from build123d import *

# Parameters (mm, degrees)
BOSS_EXTRUDE2_DEPTH     = 203.2
FILLET4_R               = 1.44
SKETCH3_R               = 1.61
SKETCH3_R_2             = 1.735
CUT_EXTRUDE2_DEPTH      = 1
CUT_EXTRUDE2_DEPTH_BACK = 16.14


with BuildPart() as part:
    # Sketch1 → Boss-Extrude2 (new body)
    with BuildSketch(Plane(origin=(0, 0, 0), x_dir=(0, 0, -1), z_dir=(1, 0, 0))):
        with BuildLine():
            Line((-10.98, 12.11), (-10.98, 1.44))
            ThreePointArc((-10.98, 1.44), (-10.558233765, 0.421766235), (-9.54, 0))
            Line((-9.54, 0), (9.54, 0))
            ThreePointArc((9.54, 0), (10.558233765, 0.421766235), (10.98, 1.44))
            Line((10.98, 1.44), (10.98, 12.11))
            ThreePointArc((10.98, 12.11), (11.401766235, 13.128233765), (12.42, 13.55))
            Line((12.42, 13.55), (18.85, 13.55))
            Line((18.85, 13.55), (18.85, 15.14))
            Line((18.85, 15.14), (10.83, 15.14))
            ThreePointArc((10.83, 15.14), (9.811766235, 14.718233765), (9.39, 13.7))
            Line((9.39, 13.7), (9.39, 3.03))
            ThreePointArc((9.39, 3.03), (8.968233765, 2.011766235), (7.95, 1.59))
            Line((7.95, 1.59), (-7.95, 1.59))
            ThreePointArc((-7.95, 1.59), (-8.968233765, 2.011766235), (-9.39, 3.03))
            Line((-9.39, 3.03), (-9.39, 13.7))
            ThreePointArc((-9.39, 13.7), (-9.811766235, 14.718233765), (-10.83, 15.14))
            Line((-10.83, 15.14), (-18.85, 15.14))
            Line((-18.85, 15.14), (-18.85, 13.55))
            Line((-18.85, 13.55), (-12.42, 13.55))
            ThreePointArc((-12.42, 13.55), (-11.401766235, 13.128233765), (-10.98, 12.11))
        make_face()
    extrude(amount=-BOSS_EXTRUDE2_DEPTH)

    # Fillet4
    fillet4_edges = [part.edges().sort_by_distance(p)[0] for p in [
        (0, 14.345, 18.85),
        (0, 14.345, -18.85),
        (-203.2, 14.345, 18.85),
        (-203.2, 14.345, -18.85),
    ]]
    fillet(fillet4_edges, radius=FILLET4_R)

    # Sketch3 → Cut-Extrude2 (cut, two sides)
    with BuildSketch(Plane(origin=(0, 15.14, 0), x_dir=(1, 0, 0), z_dir=(0, 1, 0))) as cut_extrude2_sk:
        with Locations((-101.6, 0)):
            Circle(SKETCH3_R)
        with Locations((-26.27, 0)):
            Circle(SKETCH3_R_2)
        with Locations((-176.93, 0)):
            Circle(SKETCH3_R_2)
        with Locations((-195.11, 14.89)):
            Circle(SKETCH3_R)
        with Locations((-195.11, -14.89)):
            Circle(SKETCH3_R)
        with Locations((-8.09, 14.89)):
            Circle(SKETCH3_R)
        with Locations((-8.09, -14.89)):
            Circle(SKETCH3_R)
        with BuildLine():
            Line((-137.43, -16.95), (-137.43, -18.85))
            Line((-137.43, -18.85), (-140.93, -18.85))
            Line((-140.93, -18.85), (-140.93, -16.95))
            ThreePointArc((-140.93, -16.95), (-139.18, -15.2), (-137.43, -16.95))
        make_face()
        with BuildLine():
            Line((-140.93, 18.85), (-140.93, 16.95))
            ThreePointArc((-140.93, 16.95), (-139.18, 15.2), (-137.43, 16.95))
            Line((-137.43, 16.95), (-137.43, 18.85))
            Line((-137.43, 18.85), (-140.93, 18.85))
        make_face()
        with BuildLine():
            Line((-65.77, -16.95), (-65.77, -18.85))
            Line((-65.77, -18.85), (-62.27, -18.85))
            Line((-62.27, -18.85), (-62.27, -16.95))
            ThreePointArc((-62.27, -16.95), (-64.02, -15.2), (-65.77, -16.95))
        make_face()
        with BuildLine():
            Line((-65.77, 16.95), (-65.77, 18.85))
            Line((-65.77, 18.85), (-62.27, 18.85))
            Line((-62.27, 18.85), (-62.27, 16.95))
            ThreePointArc((-62.27, 16.95), (-64.02, 15.2), (-65.77, 16.95))
        make_face()
    extrude(amount=CUT_EXTRUDE2_DEPTH, mode=Mode.SUBTRACT)
    extrude(cut_extrude2_sk.sketch, amount=-CUT_EXTRUDE2_DEPTH_BACK, mode=Mode.SUBTRACT)


solid = part.part
Verification items for the finished model (mm, model axes). A direction names the side the tool comes from. Give positions to 0.01 mm unless a question says otherwise; leave off trailing zeros. Order: outer loops, then holes, each group sorted by start corner. A loop starts at its lowest first (then second) coordinate and runs counter-clockwise, first axis right, second up. Notation, with made-up numbers: M -8.75,-24.5 L 11.25,-24.5 A19 cw 11.25,-0.5 Z; hole C 46.25,60 d8. An arc over 180 degrees is marked long. Use one line per item in the form item = value. Start each with the question number.
Q1. Mould release check, pull along X, two halves, no side actions. Record for faces 1 (the flat face through (-100, 15.14, -15)), 2 (the cylindrical face through (-196.72, 14.36, 14.82)), 3 (the flat face through (0, 1, 0)): +X half, -X half, draft (parallel to the pull), parting line (faces both ways), or undercut.
Q2. Section check B-B (x = -176.93). Enter the section's corners in (y, z) (3 decimals).
Q3. Go/stop test with flat-tipped pins: pin 1 Ø5.5 at (x, z) = (-26.27, 0) entering from +Y; pin 2 Ø5 at (x, z) = (-62, 15.5) entering from -Y; pin 3 Ø0.8 at (y, z) = (14, -18) entering from +X. Record where each tip stops, or that it passes through.
Q4. Scan lines: line 1 along X through (y, z) = (0.75, 0) (3 decimals); line 2 along X through (y, z) = (14.15, 14.89); line 3 along Z through (x, y) = (-26.27, 0.8) (3 decimals). Record each from-to range of solid material in increasing order. Write a range as [from, to].
Q5. Section check A-A (y = 8). Enter the section's corners in (x, z).
Q6. Section check C-C (x = -73). Enter the section's corners in (y, z).
Q7. Access from +Z, -Z, +X, -X, +Y, -Y to the whole of each face (thin tool, end or side, straight path). Record for faces 4 (the cylindrical face through (-7.224, 14.356, -16.248)), 5 (the flat face through (-203.2, 1, 0)), 6 (the flat face through (-100, 8, -9.39)), 7 (the flat face through (-100, 7, 10.98)), 8 (the flat face through (-100, 13.55, -16)).
Evaluation:
q1.face_1 = draft
q1.face_2 = undercut
q1.face_3 = +X half
q2.outline = M 0,-9.54 A1.44 ccw 1.44,-10.98 L 12.11,-10.98 A1.44 cw 13.55,-12.42 L 13.55,-18.85 L 15.14,-18.85 L 15.14,-10.83 A1.44 ccw 13.7,-9.39 L 3.03,-9.39 A1.44 cw 1.59,-7.95 L 1.59,-1.735 L 0,-1.735 Z; M 0,1.735 L 1.59,1.735 L 1.59,7.95 A1.44 cw 3.03,9.39 L 13.7,9.39 A1.44 ccw 15.14,10.83 L 15.14,18.85 L 13.55,18.85 L 13.55,12.42 A1.44 cw 12.11,10.98 L 1.44,10.98 A1.44 ccw 0,9.54 Z
q3.pin_1 = 1.59
q3.pin_2 = 13.55
q3.pin_3 = -0.01
q4.line_1 = [-203.2, -178.665], [-175.195, -103.21], [-99.99, -28.005], [-24.535, 0]
q4.line_2 = [-203.2, -196.72], [-193.5, -9.7], [-6.48, 0]
q4.line_3 = [-10.83, -1.735], [1.735, 10.83]
q5.outline = M -203.2,-10.98 L 0,-10.98 L 0,-9.39 L -203.2,-9.39 Z; M -203.2,9.39 L 0,9.39 L 0,10.98 L -203.2,10.98 Z
q6.outline = M 0,-9.54 A1.44 ccw 1.44,-10.98 L 12.11,-10.98 A1.44 cw 13.55,-12.42 L 13.55,-18.85 L 15.14,-18.85 L 15.14,-10.83 A1.44 ccw 13.7,-9.39 L 3.03,-9.39 A1.44 cw 1.59,-7.95 L 1.59,7.95 A1.44 cw 3.03,9.39 L 13.7,9.39 A1.44 ccw 15.14,10.83 L 15.14,18.85 L 13.55,18.85 L 13.55,12.42 A1.44 cw 12.11,10.98 L 1.44,10.98 A1.44 ccw 0,9.54 Z
q7.face_4 = +Y, -Y
q7.face_5 = +Z, -Z, -X, +Y, -Y
q7.face_6 = +X, -X, +Y
q7.face_7 = +Z, +X, -X, -Y
q7.face_8 = -Z, +X, -X, -Y
